Study the drawing (mm; zero at the part's minimum x, y, z) and answer. Coordinates: 2 decimals unless noted, no trailing zeros. Loops run counter-clockwise (first coordinate to the right, second up) from the corner with the lowest first, then second, coordinate; pieces in that order, holes last. Notation, with made-up numbers: (85, 15) - (100, 15) arc R19 cw to (100, 20) - close; hole circle Ø7 at (-33, 30). An arc over 180 degrees is marked (long way). Put each result on its own line as item: value.
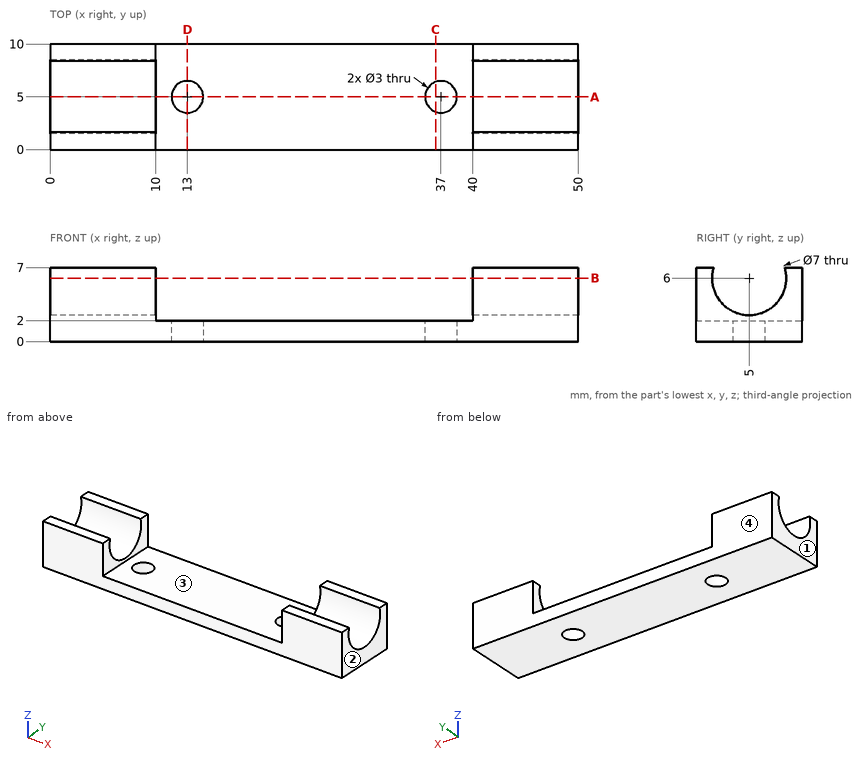
1) Straight lines are drawn through the part: L1, parallel to Y at x = 6.25, z = 6; L2, parallel to X at y = 1.25, z = 6.75; L3, parallel to Z at x = 45.5, y = 5. For each, find the intervals that lie inside material, in ascending order. Write a range as [from, to].
Found:
L1: y = [0, 1.5], [8.5, 10]
L2: x = [0, 10], [40, 50]
L3: z = [0, 2.5]
2) The part is cut by section C-C (x = 36.5). Give the vertices of the cut face in (y, z).
Found:
outline: (0, 0) - (3.59, 0) - (3.59, 2) - (0, 2) - close; (6.41, 0) - (10, 0) - (10, 2) - (6.41, 2) - close
3) For a pull along X with two mould halves and no side action, classify the marked faces 1, 2, 3 and 4 as pulls with the +X half, pulls with the -X half, needs draft (parallel to the pull), parting line crosses it, or undercut.
Found:
face 1: pulls with the -X half
face 2: pulls with the +X half
face 3: undercut
face 4: needs draft
4) Each of these flat-tipped pins is pushed along its axis until it touches: pin 1 (2.5 mm diameter, centred on x = 13, y = 5, fed in from -Z); pin 2 (4 mm diameter, centred on y = 7.5, z = 4.5, fed in from +X); pin 3 (3 mm diameter, centred on x = 27.5, y = 7, fed in from +Z). Where does it stop, or does it pass through?
Found:
pin 1: passes through
pin 2: stops at x = 50
pin 3: stops at z = 2
5) The part is cut by section A-A (y = 5). Give the vertices of the cut face in (x, z), and give its area (3 significant figures).
Found:
outline: (0, 0) - (11.5, 0) - (11.5, 2) - (10, 2) - (10, 2.5) - (0, 2.5) - close; (14.5, 0) - (35.5, 0) - (35.5, 2) - (14.5, 2) - close; (38.5, 0) - (50, 0) - (50, 2.5) - (40, 2.5) - (40, 2) - (38.5, 2) - close
area: 98.0 mm^2
6) The part is cut by section B-B (z = 6). Give the vertices of the cut face in (x, y), and give its area (3 significant figures).
Found:
outline: (0, 0) - (10, 0) - (10, 1.5) - (0, 1.5) - close; (0, 8.5) - (10, 8.5) - (10, 10) - (0, 10) - close; (40, 0) - (50, 0) - (50, 1.5) - (40, 1.5) - close; (40, 8.5) - (50, 8.5) - (50, 10) - (40, 10) - close
area: 60.0 mm^2
7) The part is cut by section D-D (x = 13). Give the vertices of the cut face in (y, z), and give its area (3 significant figures).
Found:
outline: (0, 0) - (3.5, 0) - (3.5, 2) - (0, 2) - close; (6.5, 0) - (10, 0) - (10, 2) - (6.5, 2) - close
area: 14.0 mm^2
